For this review, take the finished solid that the model builds, in its own axes (mm). Face numbers are marked on the shaded views. Coordinates: 2 decimals unless noted, no trailing zeros. Order: outer loops, then holes, each group sorted by start corner. A loop starts at its lowest first (then second) coordinate and runs counter-clockwise, first axis right, second up. Notation, with made-up numbers: (52, 66.5) -> (102, 66.5) arc R23 cw to (102, 77.5) -> close; hole circle Ø4 at (-23, -11.5). An arc over 180 degrees is marked (long way). Answer as a JSON object with one key per item and string values. Group by question number.
1) For pin 1 (3 mm diameter, centred on x = -18, y = 9, fed in from +Z); pin 2 (1.5 mm diameter, centred on x = -17, z = 11, fed in from -Y); pin 3 (1.5 mm diameter, centred on x = -16, z = 7, fed in from -Y), all flat-tipped, find the tip position at first contact; note any pin that passes through.
2) Add section A-A, the plane z = 9.75. Write out the cut boundary in (x, y).
3) Draft analysis for pull direction X (two halves, no side actions). For the marked faces 1, 2 and 3, state which applies: +X half, -X half, draft (parallel to the pull), parting line (faces both ways), or undercut.
4) Wall thickness on L1, parallel to Z at x = -20.5, y = 8; L2, parallel to X at y = 6.5, z = 8.75; L3, parallel to Y at x = -19.75, z = 12: over which ranges is each line inside the solid? List them lowest first.
from build123d import *

# Parameters (mm, degrees)
SKETCH006_R     = 4
PAD003_DEPTH    = 12
FILLET002_R     = 0.25
SKETCH007_R     = 3
POCKET003_DEPTH = 0.1


with BuildPart() as part:
    # Sketch006 (on Face1 of CopyFillet002) → Pad003 (new body)
    with BuildSketch(Plane.XY.offset(1.6)):
        with Locations((-19, 8)):
            Circle(SKETCH006_R)
    extrude(amount=PAD003_DEPTH)

    # Fillet002
    fillet002_edges = [part.edges().sort_by_distance(p)[0] for p in [
        (-23, 8, 13.6),
    ]]
    fillet(fillet002_edges, radius=FILLET002_R)

    # Sketch007 (on Face4 of Fillet002) → Pocket003 (cut)
    with BuildSketch(Plane.XY.offset(13.6)):
        with Locations((-19, 8)):
            Circle(SKETCH007_R)
    extrude(amount=-POCKET003_DEPTH, mode=Mode.SUBTRACT)


solid = part.part
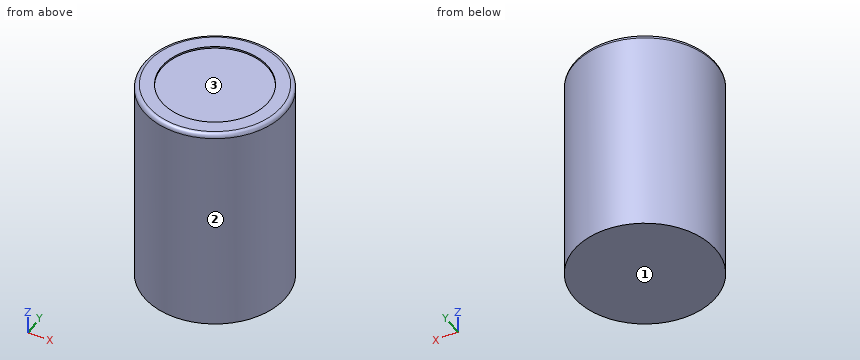
Output values:
{
 "1": {"pin 1": "stops at z = 13.5", "pin 2": "stops at y = 4.2", "pin 3": "stops at y = 4.69"},
 "2": {"outline": "circle Ø8 at (-19, 8)"},
 "3": {"face 1": "draft", "face 2": "parting line", "face 3": "undercut"},
 "4": {"L1": "z = 1.6 to 13.5", "L2": "x = -22.71 to -15.29", "L3": "y = 4.07 to 11.93"}
}
